The listing builds one solid part. Answer for the finished solid, in the listing's coordinates (mm). A direction names the side the tool comes from. Coordinates: 2 decimals unless noted, no trailing zeros. Write each loop counter-clockwise with the first axis right and the second up, starting at its lowest first coordinate (ties: lowest second). Pieces come first, ordered by that corner, then holes.
(1) Which of the six approach directions +Z, -Z, +X, -X, +Y, -Y give full straight-line access (tool end or side, diameter ignored) to faces 5 (the flat face through (-95, 79, 240)), 6 (the flat face through (-175, 79, -21.09)), 7 (the flat face through (-95, 79, -81.09)), 8 (the flat face through (350, 79, 270)), 9 (the flat face through (-110, 79, 270))?
(2) The part is cut by section D-D on x = 387. Determine the outline of the cut face in (y, z).
(3) For a pull along X with two mould halves and no side action, classify faces 1 (the flat face through (-160, 79, -52)), 2 (the flat face through (-190, 79, -51)), 3 (the flat face through (-80, 79, 270)), 4 (the flat face through (-95, 150, 270)) as +X half, -X half, draft (parallel to the pull), parting line (faces both ways), or undercut.
(4) The part is cut by section A-A on y = 55. Determine the outline of the cut face in (x, z).
(5) Straight lines are drawn through the part: line 1 (Z direction, x = -91, y = 41); line 2 (Y direction, x = 147.5, z = -62.5); line 3 (Z direction, x = 342.5, y = 31). For each, find the intervals that lie inside material, in ascending order.
(6) The part is cut by section C-C on z = -132.5. Determine the outline of the cut face in (x, y), plus the area to 3 significant figures.
(7) The part is cut by section B-B on x = 24. Determine the outline of the cut face in (y, z), plus the area to 3 significant figures.
(8) Given P1, Ø18, axis at y = 65.5, z = 274.5, coming from the -X side; P2, Ø4, axis at x = 303.5, z = 224, coming from the +Y side; P3, Ø12, axis at y = 21, z = 203, coming from the +X side; P4, Ø9, axis at x = 328, y = 70.5, coming from the -Z side, each flat-ended and moving along its own axis, determine where each tip first touches the part or whether it passes through.
Autodesk Inventor part; units mm, degrees
ref_plane "YZ Plane" through (0, 0, 0) normal (1, 0, 0) x (0, 1, 0)
ref_plane "XZ Plane" through (0, 0, 0) normal (0, 1, 0) x (-1, 0, 0)
ref_plane "XY Plane" through (0, 0, 0) normal (0, 0, 1) x (1, 0, 0)
sketch "Sketch1" plane through (0, 0, 0) normal (0, 1, 0) x (-1, 0, 0)
  line L0 (350, -300) -> (-450, -300)
  line L1 (-450, -300) -> (-450, 300)
  line L2 (-450, 300) -> (350, 300)
  line L3 (350, 300) -> (350, -300)
  line L4 (-450, 240) -> (-450, 300)
  line L5 (110, 300) -> (80, 300)
  line L6 (80, 300) -> (80, 240)
  line L7 (80, 240) -> (110, 240)
  line L8 (110, 240) -> (110, 300)
  line L9 (110, -81.09) -> (80, -81.09)
  line L10 (80, -81.09) -> (80, -21.09)
  line L11 (80, -21.09) -> (110, -21.09)
  line L12 (110, -21.09) -> (110, -81.09)
  line L13 (-320, 300) -> (-350, 300)
  line L14 (-350, 300) -> (-350, 240)
  line L15 (-350, 240) -> (-320, 240)
  line L16 (-320, 240) -> (-320, 300)
  line L17 (190, -81.09) -> (160, -81.09)
  line L18 (160, -81.09) -> (160, -21.09)
  line L19 (160, -21.09) -> (190, -21.09)
  line L20 (190, -21.09) -> (190, -81.09)
  point P0 (-50, 300)
  point P1 (350, 0)
  point P2 (95, 240)
  point P3 (80, 300)
  point P4 (110, -51.09)
  point P5 (110, 270)
  point P6 (-350, 300)
  point P7 (80, 270)
  point P8 (190, -51.09)
  dimension "d0" = 600
  dimension "d1" = 800
  dimension "d22" = 60
  dimension "d23" = 30
  dimension "d27" = 321.09
  dimension "d28" = 30
  dimension "d31" = 400
  dimension "d32" = 60
  dimension "d33" = 30
  dimension "d38" = 50
extrude "Extrusion1" add sketch "Sketch1" along normal blind 10 contours L0 L1 L2 L14 L15 L16 L6 L7 L8 L3 | L2 L16 L15 L14 | L9 L10 L11 L12 | L17 L18 L19 L20
extrude "Extrusion6" add sketch "Sketch1" along normal blind 150 contours L9 L10 L11 L12
extrude "Extrusion7" add sketch "Sketch1" along normal blind 150 contours L8 L7 L6 L2 | L2 L16 L15 L14
extrude "Extrusion8" add sketch "Sketch1" along normal blind 150 contours L17 L18 L19 L20
sketch "Sketch5" plane through (-80, 10, 240) normal (1, 0, 0) x (0, 0, -1)
  circle A0 centre (-30, 30) radius 5
  line L0 (-60, 0) -> (-60, 140)
  line L1 (-60, 0) -> (0, 0)
  point P0 (240, -10)
  dimension "d41" = 10
  dimension "d42" = 30
  dimension "d43" = 30
extrude "Extrusion9" add sketch "Sketch5" along normal up to surface (400 mm away)
equation "\"d22\" = d3"
equation "\"d23\" = d2"
equation "\"d28\" = d23"
equation "\"d32\" = d34"
equation "\"d33\" = d35"
properties part number "base"
Model answer:
1. face 5: +X, -X, +Y
1. face 6: +Z, +X, -X, +Y
1. face 7: -Z, +X, -X, +Y
1. face 8: +Z, -Z, +X, +Y
1. face 9: +Z, -Z, -X, +Y
2. outline: (0, -300) - (10, -300) - (10, 300) - (0, 300) - close
3. face 1: undercut
3. face 2: -X half
3. face 3: undercut
3. face 4: draft
4. outline: (-190, -81.09) - (-160, -81.09) - (-160, -21.09) - (-190, -21.09) - close; (-110, -81.09) - (-80, -81.09) - (-80, -21.09) - (-110, -21.09) - close; (-110, 240) - (-80, 240) - (-80, 300) - (-110, 300) - close; (320, 240) - (350, 240) - (350, 300) - (320, 300) - close
5. line 1: z = -81.09 to -21.09, 240 to 300
5. line 2: y = 0 to 10
5. line 3: z = 240 to 300
6. outline: (-350, 0) - (450, 0) - (450, 10) - (-350, 10) - close
6. area: 8,000 mm2
7. outline: (0, -300) - (10, -300) - (10, 300) - (0, 300) - close; circle Ø10 at (40, 270)
7. area: 6,080 mm2
8. P1: stops at x = -110
8. P2: stops at y = 10
8. P3: passes through
8. P4: stops at z = 240
